Geometry check sheet. Reference: drawing and pictorial views, mm from the part's lowest x, y, z. A direction names the side the tool comes from. Coordinates: 2 decimals unless noted, no trailing zeros. Write each loop counter-clockwise with the first axis right and the second up, starting at its lowest first coordinate (ties: lowest second). Pieces come first, ordered by that corner, then holes. Notation, with made-up numbers: (-1.5, 28.5) -> (22.5, 28.5) arc R30 cw to (22.5, 66.5) -> close; hole circle Ø6 at (27, 72.5). An arc over 180 degrees is marked (long way). Use a Markdown table: item, result.
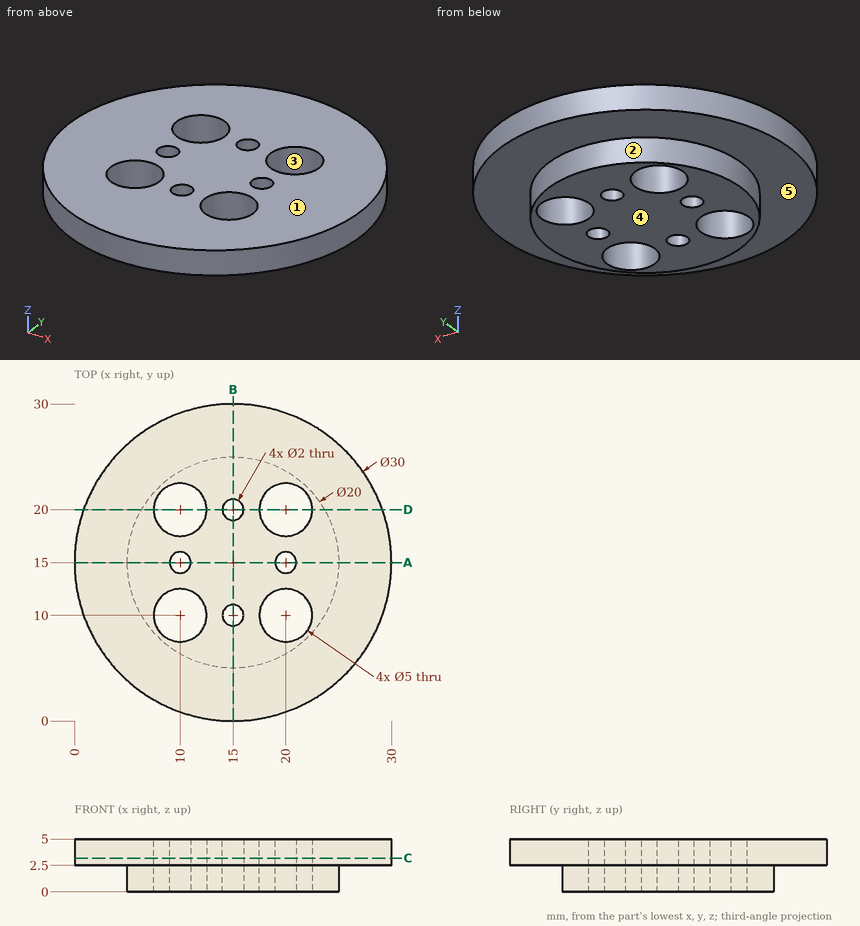
Item 1: Section check A-A on y = 15. Record the boundary of the cut face in (x, z).
Answer block:
| item | result |
|---|---|
| outline | (0, 2.5) -> (5, 2.5) -> (5, 0) -> (9, 0) -> (9, 5) -> (0, 5) -> close; (11, 0) -> (19, 0) -> (19, 5) -> (11, 5) -> close; (21, 0) -> (25, 0) -> (25, 2.5) -> (30, 2.5) -> (30, 5) -> (21, 5) -> close |
Item 2: Tool access check on the marked faces 4 and 5. Record the directions out of +Z, -Z, +X, -X, +Y, -Y that give a thin tool (end or side, any length) a straight path to the whole face; none if there is none.
Answer block:
| item | result |
|---|---|
| face 4 | -Z, +X, -X, +Y, -Y |
| face 5 | -Z |
Item 3: Mould release check, pull along X, two halves, no side actions. Record for the marked faces 1, 2 and 3: +X half, -X half, draft (parallel to the pull), parting line (faces both ways), or undercut.
Answer block:
| item | result |
|---|---|
| face 1 | draft |
| face 2 | parting line |
| face 3 | undercut |
Item 4: Depth check by flat-ended pin: P1, Ø1.5, axis at y = 18, z = 3.5, coming from the -X side; P2, Ø3, axis at x = 15, y = 10, coming from the -Z side; P3, Ø3, axis at y = 18, z = 2, coming from the +X side. Enter the tip coordinate at first touch or a pass-through.
Answer block:
| item | result |
|---|---|
| P1 | stops at x = 0.17 |
| P2 | stops at z = 0 |
| P3 | stops at x = 29.92 |
Item 5: Section check C-C on z = 3.2. Count the separate pieces of the cut face and the enclosed holes in it, then the cut area to 3 significant figures.
Answer block:
| item | result |
|---|---|
| separate pieces | 1 |
| enclosed holes | 8 |
| area | 616 mm^2 |
Item 6: Thickness scan on L1, parallel to Y at x = 15, z = 3.1; L2, parallel to Y at x = 20, z = 3.85; L3, parallel to X at y = 11.75, z = 2.8. Record the ranges inside material, lowest first. Write a range as [from, to].
Answer block:
| item | result |
|---|---|
| L1 | y = [0, 9], [11, 19], [21, 30] |
| L2 | y = [0.86, 7.5], [12.5, 14], [16, 17.5], [22.5, 29.14] |
| L3 | x = [0.36, 8.21], [11.79, 18.21], [21.79, 29.64] |
Item 7: Section check D-D on y = 20. Record the boundary of the cut face in (x, z), then the cut area to 3 significant figures.
Answer block:
| item | result |
|---|---|
| outline | (0.86, 2.5) -> (6.34, 2.5) -> (6.34, 0) -> (7.5, 0) -> (7.5, 5) -> (0.86, 5) -> close; (12.5, 0) -> (14, 0) -> (14, 5) -> (12.5, 5) -> close; (16, 0) -> (17.5, 0) -> (17.5, 5) -> (16, 5) -> close; (22.5, 0) -> (23.66, 0) -> (23.66, 2.5) -> (29.14, 2.5) -> (29.14, 5) -> (22.5, 5) -> close |
| area | 54.0 mm^2 |
